```python
from build123d import *

# Parameters (mm, degrees)
F0_R     = 31.146875323
F1_DEPTH = 6
F2_R     = 4.1697172025
F3_DEPTH = 8
F4_T     = -2.45


with BuildPart() as f1:
    # F0 (on Front) → F1 (new body)
    with BuildSketch(Plane.XZ):
        Circle(F0_R)
    extrude(amount=F1_DEPTH)

    # F2 (on face) → F3 (join)
    with BuildSketch(Plane(origin=(0, 0, 0), x_dir=(-1, 0, 0), z_dir=(0, 1, 0))):
        Circle(F2_R)
    extrude(amount=F3_DEPTH)

    # F4
    f4_openings = [f1.faces().sort_by_distance(p)[0] for p in [
        (0, 8, 0),
    ]]
    offset(amount=F4_T, openings=f4_openings, kind=Kind.INTERSECTION)


solid = f1.part
```
Here's how the part is built. I have some questions about the finished solid (model axes, mm). A direction names the side the tool comes from. Round coordinates to 2 decimals unless told otherwise and drop trailing zeros. Write each loop counter-clockwise with the first axis right and the second up, starting at its lowest first coordinate (ties: lowest second). Pieces come first, ordered by that corner, then holes. Notation, with made-up numbers: M 87,83.25 L 103,83.25 A18 cw 103,103.25 Z; hole C 51,18 d7. An arc over 180 degrees is marked long. Answer as CSV lines item,"result". Start each with the question number.
1. Suppose I cut it at C-C on x = -20.5. Write out the boundary of the cut face in (y, z), then the cut area to 3 significant figures.
2. Thinking about a two-plate mould opening in Z: for faces 4 (the cylindrical face through (-6.221, -2.992, -28.014)), 5 (the cylindrical face through (0.9, 3.94, -4.07)), 6 (the flat face through (0, -6, 0)), which applies, released by +Z, released by -Z, zero draft, split by the parting line, or undercut?
3. Suppose I cut it at A-A on z = -2.5. Write out the boundary of the cut face in (x, y).
4. Suppose I cut it at B-B on y = -1. Write out the boundary of the cut face in (x, z), then the cut area to 3 significant figures.
5. Suppose I cut it at D-D on x = 0. Write out the boundary of the cut face in (y, z).
6. I'm going to push flat-ended pins straight in: pin 1 Ø5 at (x, z) = (23, -1.5) entering from +Y; pin 2 Ø5.5 at (x, z) = (0, 0) entering from +Y; pin 3 Ø8 at (x, y) = (-23.5, -0.5) entering from +Z; pin 4 Ø2 at (y, z) = (2.5, -3) entering from +X. Where does each tip first touch, or does it pass through?
7. On a 3-axis mill with a long thin cutter (end or side, diameter ignored), from which of +Z, -Z, +X, -X, +Y, -Y can I reach the whole of each face in a straight line? I mean faces 1 (the cylindrical face through (0.37, 2.7, -1.68)), 2 (the flat face through (0, -3.55, 0)), 3 (the cylindrical face through (14.372, -2.958, -27.633)). Say none if no direction works.
8. I need wall thicknesses on probe 1 along Y at (x, z) = (21, 13.5); probe 2 along Z at (x, y) = (0, -3.2); probe 3 along Z at (x, y) = (0, 4.5). Which ranges of each line are inside material? Lowest first, please.
Check result:
1,outline,"M -6,-23.45 L 0,-23.45 L 0,23.45 L -6,23.45 Z; hole M -3.55,-20.08 L -2.45,-20.08 L -2.45,20.08 L -3.55,20.08 Z"
1,area,"237 mm2"
2,face 4,"undercut"
2,face 5,"split by the parting line"
2,face 6,"zero draft"
3,outline,"M -31.05,-6 L 31.05,-6 L 31.05,0 L 3.34,0 L 3.34,8 L -3.34,8 L -3.34,0 L -31.05,0 Z; hole M -28.59,-3.55 L 28.59,-3.55 L 28.59,-2.45 L -28.59,-2.45 Z"
4,outline,"C 0,0 d62.29; hole C 0,0 d3.44"
4,area,"3,040 mm2"
5,outline,"M -6,-31.15 L 0,-31.15 L 0,-4.17 L 8,-4.17 L 8,-1.72 L -2.45,-1.72 L -2.45,-28.7 L -3.55,-28.7 L -3.55,28.7 L -2.45,28.7 L -2.45,1.72 L 8,1.72 L 8,4.17 L 0,4.17 L 0,31.15 L -6,31.15 Z"
6,pin 1,"stops at y = 0"
6,pin 2,"stops at y = 8"
6,pin 3,"stops at z = 24.29"
6,pin 4,"stops at x = 3.66"
7,face 1,"+Y"
7,face 2,"none"
7,face 3,"+Y, -Y"
8,probe 1,"y = -6 to -3.55, -2.45 to 0"
8,probe 2,"z = -31.15 to -28.7, 28.7 to 31.15"
8,probe 3,"z = -4.17 to -1.72, 1.72 to 4.17"
